The model under review builds one solid part; all positions refer to its coordinate system, in mm. Round coordinates to 2 decimals unless told otherwise and drop trailing zeros. Loops run counter-clockwise (first coordinate to the right, second up) from the corner with the lowest first, then second, coordinate; pieces in that order, holes last. Notation, with made-up numbers: (21.25, 71) -> (29.25, 71) arc R20 ccw to (29.25, 99) -> close; hole circle Ø5 at (79.25, -9.75). An arc over 180 degrees is marked (long way). Use a Markdown table: item, result. Add a question column.
1) Consider section A-A on x = 20.5. Give the boundary of the cut face in (y, z).
2) Consider section C-C on z = -2.25. Give the boundary of the cut face in (x, y), plus the area to 3 significant figures.
3) Insertion check: pin 1 (2 mm diameter, centred on x = 13.5, y = 12.5, fed in from +Z); pin 2 (4 mm diameter, centred on x = 13.5, z = 1.5, fed in from -Y); pin 3 (2 mm diameter, centred on y = 9, z = -1, fed in from +X). Each pin has a flat end and moves straight along its axis. Give the tip position at first contact, or say it passes through.
4) Consider section B-B on z = 1.25. Give the boundary of the cut face in (x, y).
5) Mouldability with a two-part tool opening along Y and no side actions: class faces 1 (the cylindrical face through (20.723, 10.198, 1.972)), 2 (the flat face through (15, 12, 3)), 3 (the flat face through (21, 14, 0)) as released by +Y, released by -Y, zero draft, split by the parting line, or undercut.
6) Wall thickness on probe 1 along Z at (x, y) = (9, 9.5); probe 2 along Z at (x, y) = (15, 13.5); probe 3 along X at (y, z) = (9.75, 3.5): over which ranges is each line inside the solid? List them lowest first.
Autodesk Inventor part; units mm, degrees
ref_plane "YZ Plane" through (0, 0, 0) normal (1, 0, 0) x (0, 1, 0)
ref_plane "XZ Plane" through (0, 0, 0) normal (0, 1, 0) x (-1, 0, 0)
ref_plane "XY Plane" through (0, 0, 0) normal (0, 0, 1) x (1, 0, 0)
sketch "Sketch1" plane through (0, 0, 0) normal (0, 0, 1) x (1, 0, 0)
  circle A0 centre (15, 12) radius 6
  circle A1 centre (15, 12) radius 7
  point P0 (0, 0)
  dimension "d0" = 12
  dimension "d1" = 14
extrude "Extrusion1" add sketch "Sketch1" along normal blind 4 contours A0
extrude "Extrusion2" add sketch "Sketch1" against normal blind 3 contours A0 | A1
sketch "Sketch2" plane through (15, 12, 4) normal (0, 0, 1) x (1, 0, 0)
  circle A0 centre (0, 0) radius 5
  point P0 (-15, -12)
  dimension "d6" = 10
extrude "Extrusion3" cut sketch "Sketch2" against normal blind 1
fillet "Fillet1" radius 5 1 edges at (10, 12, 3)
properties part number "but"
Result set:
| question | item | result |
|---|---|---|
| 1 | outline | (7.67, -3) -> (16.33, -3) -> (16.33, 0) -> (14.4, 0) -> (14.4, 4) -> (9.6, 4) -> (9.6, 0) -> (7.67, 0) -> close |
| 2 | outline | circle Ø14 at (15, 12) |
| 2 | area | 154 mm2 |
| 3 | pin 1 | z = 3.03 |
| 3 | pin 2 | y = 5 |
| 3 | pin 3 | x = 21.71 |
| 4 | outline | circle Ø12 at (15, 12) |
| 5 | face 1 | split by the parting line |
| 5 | face 2 | undercut |
| 5 | face 3 | zero draft |
| 6 | probe 1 | -3 to 0 |
| 6 | probe 2 | -3 to 3 |
| 6 | probe 3 | 9.44 to 11.48, 18.52 to 20.56 |
